```python
from build123d import *

# Parameters (mm, degrees)
F0_R     = 35
F0_R_2   = 10.5
F1_DEPTH = 5
F0_R_3   = 8
F2_DEPTH = 70
F3_DEPTH = 65


with BuildPart() as f1:
    # F0 (on Top) → F1 (new body)
    with BuildSketch(Plane.XY):
        Circle(F0_R)
        Circle(F0_R_2, mode=Mode.SUBTRACT)
    extrude(amount=F1_DEPTH)

    # F0 (on Top) → F2 (join)
    with BuildSketch(Plane.XY):
        Circle(F0_R_2)
        Circle(F0_R_3, mode=Mode.SUBTRACT)
    extrude(amount=F2_DEPTH)

    # F0 (on Top) → F3 (join)
    with BuildSketch(Plane.XY):
        Circle(F0_R_3)
    extrude(amount=F3_DEPTH)


solid = f1.part
```
Verification items for the finished model (mm, model axes). A direction names the side the tool comes from. Coordinates: 2 decimals unless noted, no trailing zeros. Write each loop counter-clockwise with the first axis right and the second up, starting at its lowest first coordinate (ties: lowest second). Pieces come first, ordered by that corner, then holes. Notation, with made-up numbers: M 50.5,37 L 61.5,37 A13 cw 61.5,45 Z; hole C 50,-37.75 d2. An arc over 180 degrees is marked long. One line per item, written item: value.
Item 1: Gauge pin test, flat ends, axial feed: pin 1 Ø12 at (x, z) = (-10.5, 15) entering from +Y; pin 2 Ø2 at (y, z) = (-1.5, 25) entering from -X; pin 3 Ø10 at (x, y) = (20.5, -12) entering from +Z. Record the tip position at first contact, or that the pin passes through.
Check sheet entries:
pin 1: stops at y = 9.49
pin 2: stops at x = -10.49
pin 3: stops at z = 5
Item 2: Scan lines: line 1 along Y through (x, z) = (0, 67); line 2 along Z through (x, y) = (-12.5, 28); line 3 along Z through (x, y) = (6, -4). Record each from-to range of solid material in increasing order.
Check sheet entries:
line 1: y = -10.5 to -8, 8 to 10.5
line 2: z = 0 to 5
line 3: z = 0 to 65
Item 3: Mould release check, pull along X, two halves, no side actions. Record for faces 1 (the flat face through (0, 0, 65)), 2 (the flat face through (-2, -8, 70)), 3 (the cylindrical face through (-28, -21, 2)), 4 (the cylindrical face through (-1.73, -7.81, 67.46)): pulls with the +X half, pulls with the -X half, needs draft (parallel to the pull), parting line crosses it, or undercut.
Check sheet entries:
face 1: undercut
face 2: needs draft
face 3: parting line crosses it
face 4: undercut
Item 4: Access from +Z, -Z, +X, -X, +Y, -Y to the whole of each face (thin tool, end or side, straight path). Record for faces 5 (the cylindrical face through (10, 3.2, 37)), 6 (the flat face through (0, 0, 0)).
Check sheet entries:
face 5: +Z
face 6: -Z, +X, -X, +Y, -Y
Item 5: Section check C-C, the plane z = 26. Record the boundary of the cut face in (x, y), plus the area to 3 significant figures.
Check sheet entries:
outline: C 0,0 d21
area: 346 mm^2
Item 6: Section check B-B, the plane x = -1. Record the boundary of the cut face in (y, z), plus the area to 3 significant figures.
Check sheet entries:
outline: M -34.99,0 L 34.99,0 L 34.99,5 L 10.45,5 L 10.45,70 L 7.94,70 L 7.94,65 L -7.94,65 L -7.94,70 L -10.45,70 L -10.45,5 L -34.99,5 Z
area: 1,630 mm^2
Item 7: Section check D-D, the plane y = 13.5. Record the boundary of the cut face in (x, z), plus the area to 3 significant figures.
Check sheet entries:
outline: M -32.29,0 L 32.29,0 L 32.29,5 L -32.29,5 Z
area: 323 mm^2
Item 8: Section check A-A, the plane y = 0. Record the boundary of the cut face in (x, z).
Check sheet entries:
outline: M -35,0 L 35,0 L 35,5 L 10.5,5 L 10.5,70 L 8,70 L 8,65 L -8,65 L -8,70 L -10.5,70 L -10.5,5 L -35,5 Z
